Model file for the job. Use its own axes, mm. A direction names the side the tool comes from. Round coordinates to 2 decimals unless told otherwise and drop trailing zeros. Write each loop counter-clockwise with the first axis right and the second up, starting at its lowest first coordinate (ties: lowest second). Pieces come first, ordered by that corner, then holes. Notation, with made-up numbers: (3, 20) - (29, 20) arc R8 ccw to (29, 33) - close; hole circle Ø10 at (14.25, 70.25). An arc over 180 degrees is marked (long way). Answer as a JSON object with one key per item and string values. Group by question number.
Autodesk Inventor part; units mm, degrees
ref_plane "YZ Plane" through (0, 0, 0) normal (1, 0, 0) x (0, 1, 0)
ref_plane "XZ Plane" through (0, 0, 0) normal (0, 1, 0) x (-1, 0, 0)
ref_plane "XY Plane" through (0, 0, 0) normal (0, 0, 1) x (1, 0, 0)
sketch "Sketch1" plane through (0, 0, 0) normal (0, 0, 1) x (1, 0, 0)
  line L0 (12.2, 0) -> (64.2, 0)
  line L1 (64.2, 0) -> (64.2, 72)
  line L2 (64.2, 72) -> (0, 72)
  line L3 (0, 72) -> (0, 12)
  line L4 (3, 66) -> (9.5, 66)
  line L5 (9.5, 66) -> (9.5, 58)
  line L6 (9.5, 58) -> (3, 58)
  line L7 (3, 58) -> (3, 66)
  line L8 (3, 43) -> (9.5, 43)
  line L9 (9.5, 43) -> (9.5, 35)
  line L10 (9.5, 35) -> (3, 35)
  line L11 (3, 35) -> (3, 43)
  line L12 (0, 12) -> (12.2, 12)
  line L13 (12.2, 12) -> (12.2, 0)
  line L14 (3, 58) -> (9.5, 43) construction
  line L15 (3, 43) -> (9.5, 58) construction
  circle A0 centre (6.25, 50.5) radius 2.25
  point P0 (0, 0)
  dimension "d1" = 6.5
  dimension "d2" = 8
  dimension "d3" = 8
  dimension "d4" = 15
  dimension "d5" = 3
  dimension "d6" = 72
  dimension "d7" = 4.5
  dimension "d8" = 64.2
  dimension "d9" = 12
  dimension "d10" = 52
  dimension "d11" = 6
extrude "Extrusion1" add sketch "Sketch1" along normal blind 6.5
sketch "Sketch2" plane through (0, 0, 6.5) normal (0, 0, 1) x (1, 0, 0)
  line L0 (64.2, 0) -> (64.2, 72)
  line L1 (12.2, 0) -> (64.2, 0)
  line L2 (29.95, 16.3) -> (34.45, 16.3)
  line L3 (34.45, 0) -> (29.95, 0)
  line L4 (36.95, 12.3) -> (36.95, 5)
  line L5 (27.45, 5) -> (27.45, 12.3)
  line L6 (29.95, 0) -> (29.95, 5)
  line L7 (29.95, 12.3) -> (29.95, 16.3)
  line L8 (27.45, 12.3) -> (29.95, 12.3)
  line L9 (34.45, 12.3) -> (36.95, 12.3)
  line L10 (34.45, 16.3) -> (34.45, 12.3)
  line L11 (34.45, 5) -> (34.45, 0)
  line L12 (36.95, 5) -> (34.45, 5)
  line L13 (29.95, 5) -> (27.45, 5)
  point P0 (0, 0)
  point P1 (32.2, 16.3)
  dimension "d14" = 2.5
  dimension "d15" = 2.5
  dimension "d16" = 4.5
  dimension "d17" = 5
  dimension "d18" = 7.3
  dimension "d19" = 4
  dimension "d20" = 32
extrude "Extrusion2" cut sketch "Sketch2" against normal blind 6.5
sketch "Sketch3" plane through (0, 0, 6.5) normal (0, 0, 1) x (1, 0, 0)
  line L0 (34.45, 0) -> (64.2, 0)
  line L1 (12.2, 0) -> (29.95, 0)
  line L2 (29.95, 16.3) -> (34.45, 16.3)
  line L3 (16.7, 0) -> (24.7, 0)
  line L4 (24.7, 0) -> (24.7, -4.5)
  line L5 (22.7, -6.5) -> (18.7, -6.5)
  line L6 (16.7, -4.5) -> (16.7, 0)
  line L7 (39.7, 0) -> (47.7, 0)
  line L8 (47.7, 0) -> (47.7, -4.5)
  line L9 (45.7, -6.5) -> (41.7, -6.5)
  line L10 (39.7, -4.5) -> (39.7, 0)
  arc A0 (16.7, -4.5) -> (18.7, -6.5) centre (18.7, -4.5) ccw
  arc A1 (22.7, -6.5) -> (24.7, -4.5) centre (22.7, -4.5) ccw
  arc A2 (39.7, -4.5) -> (41.7, -6.5) centre (41.7, -4.5) ccw
  arc A3 (45.7, -6.5) -> (47.7, -4.5) centre (45.7, -4.5) ccw
  point P0 (0, 0)
  point P1 (32.2, 16.3)
  dimension "d23" = 2
  dimension "d24" = 8
  dimension "d25" = 8
  dimension "d26" = 6.5
  dimension "d27" = 15
  dimension "d28" = 7.5
extrude "Extrusion3" add sketch "Sketch3" against normal blind 6.5
chamfer "Chamfer1" distance 2 angle 45 2 edges at (0, 72, 3.25) (64.2, 72, 3.25)
sketch "Sketch4" plane through (0, 0, 0) normal (0, 0, -1) x (-1, 0, 0)
  line L0 (-64.2, 70) -> (-64.2, 0)
  line L1 (-2, 72) -> (-62.2, 72)
  line L2 (-39.2, 59) -> (-53.2, 59)
  line L3 (-53.2, 59) -> (-53.2, 45)
  line L4 (-53.2, 45) -> (-39.2, 45)
  line L5 (-39.2, 45) -> (-39.2, 59)
  line L6 (-34.2, 66) -> (-58.2, 66) construction
  line L7 (-58.2, 66) -> (-58.2, 38) construction
  line L8 (-58.2, 38) -> (-34.2, 38) construction
  line L9 (-34.2, 38) -> (-34.2, 66) construction
  circle A0 centre (-58.2, 61) radius 1.6
  circle A1 centre (-58.2, 43) radius 1.6
  circle A2 centre (-53.2, 38) radius 1.6
  circle A3 centre (-39.2, 38) radius 1.6
  circle A4 centre (-34.2, 43) radius 1.6
  circle A5 centre (-34.2, 61) radius 1.6
  circle A6 centre (-39.2, 66) radius 1.6
  circle A7 centre (-53.2, 66) radius 1.6
  point P0 (0, 0)
  point P1 (-58.2, 52)
  point P2 (-53.2, 52)
  point P3 (-46.2, 38)
  point P4 (-46.2, 45)
  dimension "d34" = 3.2
  dimension "d35" = 5
  dimension "d36" = 5
  dimension "d37" = 5
  dimension "d38" = 5
  dimension "d39" = 5
  dimension "d40" = 5
  dimension "d41" = 5
  dimension "d42" = 5
  dimension "d43" = 14
  dimension "d44" = 14
  dimension "d45" = 5
  dimension "d46" = 7
  dimension "d47" = 6
  dimension "d48" = 6
extrude "Extrusion4" cut sketch "Sketch4" against normal through all
chamfer "Chamfer2" distance 2 angle 45 2 edges at (0, 12, 3.25) (12.2, 12, 3.25)
equation "\"d36\" = d35"
equation "\"d37\" = d35"
equation "\"d38\" = d35"
equation "\"d39\" = d35"
equation "\"d40\" = d35"
equation "\"d41\" = d35"
equation "\"d42\" = d35"
properties part number "x_motor_cable_mount"
(1) Pull direction Y, two halves, no side cores. Call faces 1 (the flat face through (6, 58, 3)), 2 (the flat face through (24.7, -2, 3)), 3 (the cylindrical face through (40.27, -5.9, 3.3)): pulls with the +Y half, pulls with the -Y half, needs draft (parallel to the pull), parting line crosses it, or undercut.
(2) 3-axis set-ups, long thin cutter, end or side, ignore diameter. For faces 4 (the flat face through (0, 42, 3)), 5 (the flat face through (39.7, -2, 3)), 6 (the flat face through (12.2, 5, 3)), 7 (the flat face through (53.2, 52, 3)): which of +Z, -Z, +X, -X, +Y, -Y reach the whole face in a straight line?
(3) Flat gauge pins, fed straight in: pin 1 (3.5 mm diameter, centred on y = -3, z = 3.5, fed in from +X); pin 2 (2 mm diameter, centred on y = -2, z = 4.5, fed in from -X); pin 3 (1.3 mm diameter, centred on x = 14.5, z = 3.5, fed in from -Y); pin 4 (3 mm diameter, centred on x = 34.2, y = 61, fed in from +Z). Where does each tip first touch, or does it go through?
(4) Slice it at A-A (x = 43). Write the cut outline in (y, z), then the cut area to 3 significant figures.
(5) Slice it at B-B (y = 61). Write the cut outline in (x, z), then the cut area to 3 significant figures.
(6) Slice it at D-D (y = 50.5). Write the cut outline in (x, z).
(7) Drill centre lines: line 1 (Y direction, x = 58.2, z = 2.25); line 2 (X direction, y = 64, z = 5.25); line 3 (Y direction, x = 50, z = 1). Where is each one in solid material? Low to high. Write a range as from..to.
(8) Slice it at C-C (x = 58.2). Write the cut outline in (y, z).
Answer:
{
 "1": {"face 1": "undercut", "face 2": "needs draft", "face 3": "pulls with the -Y half"},
 "2": {"face 4": "+Z, -Z, -X, +Y, -Y", "face 5": "+Z, -Z, -Y", "face 6": "+Z, -Z, -X, -Y", "face 7": "+Z, -Z"},
 "3": {"pin 1": "x = 47.7", "pin 2": "x = 16.7", "pin 3": "y = 0", "pin 4": "through"},
 "4": {"outline": "(-6.5, 0) - (45, 0) - (45, 6.5) - (-6.5, 6.5) - close; (59, 0) - (72, 0) - (72, 6.5) - (59, 6.5) - close", "area": "419 mm²"},
 "5": {"outline": "(0, 0) - (3, 0) - (3, 6.5) - (0, 6.5) - close; (9.5, 0) - (32.6, 0) - (32.6, 6.5) - (9.5, 6.5) - close; (35.8, 0) - (56.6, 0) - (56.6, 6.5) - (35.8, 6.5) - close; (59.8, 0) - (64.2, 0) - (64.2, 6.5) - (59.8, 6.5) - close", "area": "333 mm²"},
 "6": {"outline": "(0, 0) - (4, 0) - (4, 6.5) - (0, 6.5) - close; (8.5, 0) - (39.2, 0) - (39.2, 6.5) - (8.5, 6.5) - close; (53.2, 0) - (64.2, 0) - (64.2, 6.5) - (53.2, 6.5) - close"},
 "7": {"line 1": "0..41.4, 44.6..59.4, 62.6..72", "line 2": "0..3, 9.5..64.2", "line 3": "0..45, 59..72"},
 "8": {"outline": "(0, 0) - (41.4, 0) - (41.4, 6.5) - (0, 6.5) - close; (44.6, 0) - (59.4, 0) - (59.4, 6.5) - (44.6, 6.5) - close; (62.6, 0) - (72, 0) - (72, 6.5) - (62.6, 6.5) - close"}
}
